Geometry: final body of the model. Coordinates: model frame, mm. A direction names the side the tool comes from. Round coordinates to 2 decimals unless told otherwise and drop trailing zeros. Write each loop counter-clockwise with the first axis right and the second up, starting at its lowest first coordinate (ties: lowest second). Pieces come first, ordered by that corner, then holes. Notation, with made-up numbers: (-19.5, -14.5) -> (34.5, -14.5) arc R12 ccw to (34.5, -6.5) -> close; hole circle Ø5 at (-1, -27.75). An arc over 180 degrees is marked (long way). One line per item, written item: value. Start each with the question number.
from build123d import *

# Parameters (mm, degrees)
BOSS_EXTRUDE1_DEPTH = 10
SKETCH2_R           = 7.5
BOSS_EXTRUDE4_DEPTH = 10
SKETCH3_R           = 7.5
CUT_EXTRUDE1_DEPTH  = 60
SKETCH4_R           = 3
CUT_EXTRUDE2_DEPTH  = 60
FILLET1_R           = 2


with BuildPart() as part:
    # Sketch1 → Boss-Extrude1 (new, symmetric)
    with BuildSketch(Plane.XY):
        with BuildLine():
            Line((-38.1, 0), (-25.4, 0))
            ThreePointArc((-25.4, 0), (0, 25.4), (25.4, 0))
            Line((25.4, 0), (38.1, 0))
            ThreePointArc((38.1, 0), (0, 38.1), (-38.1, 0))
        make_face()
    extrude(amount=BOSS_EXTRUDE1_DEPTH, both=True)

    # Sketch2 → Boss-Extrude4 (add)
    with BuildSketch(Plane.XZ):
        with Locations((38.1, 0)):
            Circle(SKETCH2_R)
    boss_extrude4 = extrude(amount=-BOSS_EXTRUDE4_DEPTH)

    # Sketch3 → Cut-Extrude1 (cut)
    with BuildSketch(Plane(origin=(0, 10, 0), x_dir=(1, 0, 0), z_dir=(0, 1, 0))):
        with Locations((38.1, 0)):
            Circle(SKETCH3_R)
    cut_extrude1 = extrude(amount=CUT_EXTRUDE1_DEPTH, mode=Mode.SUBTRACT)

    # Sketch4 → Cut-Extrude2 (cut)
    with BuildSketch(Plane.XZ):
        with Locations(Location((38.1, 0, 0), (0, 0, 270))):
            Circle(SKETCH4_R)
    cut_extrude2 = extrude(amount=-CUT_EXTRUDE2_DEPTH, mode=Mode.SUBTRACT)

    # Mirror1: Boss-Extrude4, Cut-Extrude1, Cut-Extrude2 across plane
    add(boss_extrude4.mirror(Plane(origin=(0, 0, 0), x_dir=(0, 0, 1), z_dir=(1, 0, 0))))
    add(cut_extrude1.mirror(Plane(origin=(0, 0, 0), x_dir=(0, 0, 1), z_dir=(1, 0, 0))), mode=Mode.SUBTRACT)
    add(cut_extrude2.mirror(Plane(origin=(0, 0, 0), x_dir=(0, 0, 1), z_dir=(1, 0, 0))), mode=Mode.SUBTRACT)

    # Fillet1
    fillet1_edges = [part.edges().sort_by_distance(p)[0] for p in [
        (0, 38.1, 10),
        (0, 25.4, 10),
        (0, 38.1, -10),
        (0, 25.4, -10),
    ]]
    fillet(fillet1_edges, radius=FILLET1_R)


solid = part.part
(1) Pull-direction query (X, two-part tool) for faces 1 (the face through (-0.559, 25.394, 0.112)), 2 (the face through (-41.3, 10, 0.1)), 3 (the face through (-30.6, 14.8, -0.1)); classes: pulls with the +X half, pulls with the -X half, needs draft (parallel to the pull), parting line crosses it, or undercut.
(2) Line query: probe 1 along Z at (x, y) = (-38.1, 4.25); probe 2 along X at (y, z) = (5.5, 0); probe 3 along X at (y, z) = (5.5, -2.5). Output: solid intervals per line, ascending.
(3) Set-up query: faces 4 (the face through (41.3, 10, 0.1)), 5 (the face through (0, 29, -10)). Return all of +Z, -Z, +X, -X, +Y, -Y with unobstructed straight access to the full face (end or side cutting, diameter ignored); none if empty.
(4) Section query B-B (x = 0). Output: boundary loops of the cut face in (y, z).
(5) Pin query (flat end, axial travel): pin 1 (10 mm diameter, centred on x = 2, z = 2, fed in from +Y); pin 2 (10 mm diameter, centred on x = 24, y = 34, fed in from -Z); pin 3 (5 mm diameter, centred on y = 29, z = 2, fed in from +X); pin 4 (10 mm diameter, centred on x = -4, y = 22.5, fed in from -Z). Return the tip coordinate at first contact, or that it passes through.
(6) Section query A-A (z = 0). Output: boundary loops of the cut face in (x, y).
Results list:
1. face 1: undercut
1. face 2: needs draft
1. face 3: pulls with the -X half
2. probe 1: z = -7.5 to -3, 3 to 7.5
2. probe 2: x = -45.6 to -41.1, -35.1 to -24.8, 24.8 to 35.1, 41.1 to 45.6
2. probe 3: x = -45.17 to -39.76, -36.44 to -24.8, 24.8 to 36.44, 39.76 to 45.17
3. face 4: +X, +Y
3. face 5: -Z, +X, -X, +Y, -Y
4. outline: (25.4, -8) arc R2 ccw to (27.4, -10) -> (36.1, -10) arc R2 ccw to (38.1, -8) -> (38.1, 8) arc R2 ccw to (36.1, 10) -> (27.4, 10) arc R2 ccw to (25.4, 8) -> close
5. pin 1: stops at y = 38.1
5. pin 2: stops at z = -9.93
5. pin 3: stops at x = 27.37
5. pin 4: stops at z = -10
6. outline: (-45.6, 0) -> (-41.1, 0) -> (-41.1, 10) -> (-45.6, 10) -> close; (-35.1, 0) -> (-25.4, 0) arc R25.4 cw to (25.4, 0) -> (35.1, 0) -> (35.1, 10) -> (30.6, 10) -> (30.6, 22.7) arc R38.1 ccw to (-30.6, 22.7) -> (-30.6, 10) -> (-35.1, 10) -> close; (41.1, 0) -> (45.6, 0) -> (45.6, 10) -> (41.1, 10) -> close
